Work out the finished part from the listing and answer in its coordinate system (mm). A direction names the side the tool comes from. Coordinates: 2 decimals unless noted, no trailing zeros. Order: outer loops, then holes, each group sorted by start corner. A loop starts at its lowest first (then second) coordinate and runs counter-clockwise, first axis right, second up. Notation, with made-up numbers: M -26,-16 L -14,-16 A17 cw -14,12 Z; hole C 74.25,-29 d9. An arc over 180 degrees is marked long. Answer in a Markdown table with one row per item. Add a question column.
Item 1: The part is cut by section B-B (x = 0). State how many separate pieces and enclosed holes the cut face has, then the cut area to 3 significant figures.
Item 2: Flat-ended cylindrical pins translate along their axes: pin 1 Ø0.8 at (x, y) = (0.5, 0) entering from +Z; pin 2 Ø2.5 at (x, z) = (-2.5, 1.5) entering from -Y; pin 3 Ø0.5 at (x, z) = (0.5, 19) entering from +Y; pin 4 Ø1 at (x, z) = (0, 19.32) entering from +Y. Find the tip coordinate at first contact, or state that the pin passes through.
Item 3: Consider line 1 (Y direction, x = 0, z = 16.2) (3 decimals); line 2 (Z direction, x = 0, y = 1); line 3 (Z direction, x = 0, y = 32.35). Determine where each line is inside the solid, lowest interval first. Write a range as from..to.
Item 4: Which of the six approach directions +Z, -Z, +X, -X, +Y, -Y give full straight-line access (tool end or side, diameter ignored) to faces 1 (the face through (-0.925, -0.5, -0.2)), 2 (the face through (0, 0.7, 13)), 3 (the face through (0, 15, 13.824)), 4 (the face through (0.925, -0.5, -0.2))?
Item 5: The mould has two halves that part along X. Classify faces 5 (the face through (-3.05, 2, 8)), 6 (the face through (0, 33.5, 18)), 7 (the face through (0.1, 1.17, 2.23)): released by +X, released by -X, zero draft, split by the parting line, or undercut.
Item 6: The part is cut by section C-C (y = 2). Write down the section's boundary in (x, z), then the cut area to 3 significant figures.
Item 7: The part is cut by section D-D (z = 10). Write down the section's boundary in (x, y).
Item 8: The part is cut by section A-A (z = -2.5). Write down the section's boundary in (x, y) (3 decimals), then the cut area to 3 significant figures.
Autodesk Inventor part; units mm, degrees
ref_plane "Work Plane3" through (-3.05, 3.4, 13.8245) normal (0, 0, 1) x (1, 0, 0)
ref_plane "YZ Plane" through (0, 0, 0) normal (1, 0, 0) x (0, 1, 0)
ref_plane "XZ Plane" through (0, 0, 0) normal (0, 1, 0) x (-1, 0, 0)
sketch "Sketch1" plane through (0, 0, 0) normal (0, 1, 0) x (-1, 0, 0)
  line L0 (3.05, -5.3255) -> (-3.05, -5.3255)
  line L1 (-3.05, -5.3255) -> (-3.05, 4.8245)
  line L2 (-3.05, 4.8245) -> (3.05, 4.8245)
  line L3 (3.05, 4.8245) -> (3.05, -5.3255)
  line L4 (0.925, 4.8245) -> (-0.925, 4.8245)
  line L5 (0.925, 4.8245) -> (0.925, -5.3255)
  line L6 (-0.925, 4.8245) -> (-0.925, -5.3255)
  circle A0 centre (0, 3.0245) radius 0.8
  circle A1 centre (0, -3.8255) radius 0.8
  line L7 (0, 4.8245) -> (0, -5.3255)
  line L8 (-3.05, 0) -> (3.05, 0)
  point P0 (0, 0)
  dimension "d13" = 6.1
  dimension "d44" = 1.85
  dimension "d45" = 2.125
  dimension "d46" = 1.6
  dimension "d47" = 1.6
  dimension "d128" = 6.85
extrude "Extrusion1" add sketch "Sketch1" along normal blind 3.4 contours L0 L5 L8 L3 | L0 L7 A1 L8 L5 | L8 L5 L2 L3 | L0 L6 L8 L7 A1 | L8 L7 A0 L2 L5 | L0 L1 L8 L6 | L8 L6 L2 L7 A0 | L8 L1 L2 L6
extrude "Extrusion6" add sketch "Sketch1" against normal blind 1 contours L0 L7 A1 L8 L5 | L0 L6 L8 L7 A1 | L8 L7 A0 L2 L5 | L8 L6 L2 L7 A0
sketch "Sketch13" plane through (-3.05, 3.4, 4.8245) normal (0, 0, 1) x (1, 0, 0)
  line L0 (0, 0) -> (0, -2.7)
  line L1 (0, -3.4) -> (0, 0)
  line L2 (0, -2.7) -> (6.1, -2.7)
  line L3 (6.1, -3.4) -> (6.1, 0)
  line L4 (6.1, 0) -> (6.1, -2.7)
  line L5 (0, 0) -> (6.1, 0)
  point P0 (3.05, -3.4)
  point P1 (6.1, -3.41)
  dimension "d56" = 2.7
extrude "Extrusion8" add sketch "Sketch13" along normal blind 17
sketch "Sketch17" plane through (-3.05, 3.4, 21.8245) normal (0, 0, 1) x (1, 0, 0)
  line L0 (6.1, 0) -> (0, 0)
  line L1 (6.1, 0) -> (19.567, 0) construction
  line L2 (16.968, 8.2706) -> (10.0894, 18.4685)
  line L3 (10.0894, 18.4685) -> (13.5713, 20.8172)
  line L4 (13.5713, 20.8172) -> (20.102, 11.1351)
  line L5 (20.102, 11.1351) -> (22.1374, 8.1174)
  line L6 (6.1, -3.4) -> (6.1, -2.7)
  line L7 (22.1374, 8.1174) -> (6.1, -2.7)
  line L8 (6.1, 0) -> (6.1, -2.7)
  line L9 (6.1, 0.94) -> (6.1, 0)
  line L10 (6.1, 0.94) -> (3.05, 0.94)
  line L11 (3.05, 0.94) -> (3.05, 0)
  line L12 (16.968, 8.2706) -> (6.1, 0.94)
  line L13 (6.1, 0.94) -> (7.7497, 0.94)
  point P0 (3.05, -3.4)
  dimension "d74" = 12.301
  dimension "d75" = 4.2
  dimension "d92" = 3.64
  dimension "d93" = 3.64
  dimension "d94" = 10.868
  dimension "d98" = 34
extrude "Extrusion12" [suppressed]
ref_plane "Work Plane3" through (-3.05, 3.4, 13.8245) normal (0, 0, 1) x (1, 0, 0)
sketch "Sketch29" plane through (-3.05, 3.4, 13.8245) normal (0, 0, 1) x (1, 0, 0)
  line L0 (3.85, -4.4) -> (2.25, -4.4)
  line L1 (3.05, -4.4) -> (3.05, 30.1)
  line L2 (4.95, 30.1) -> (3.05, 30.1)
  line L3 (3.05, 30.1) -> (1.15, 30.1)
  line L4 (6.1, -3.4) -> (6.1, 0)
  line L5 (4.95, 30.1) -> (6.1, 0)
  line L6 (0, -3.4) -> (0, 0)
  line L7 (1.15, 30.1) -> (0, 0)
  line L8 (0, 0) -> (6.1, 0)
  point P0 (3.05, -3.4)
  point P1 (3.0506, 28.6)
  dimension "d137" = 34.5
  dimension "d138" = 3.8
extrude "Extrusion20" add sketch "Sketch29" along normal blind 8
fillet "Fillet6" radius 0.5 2 edges at (2.475, 18.45, 13.8245) (-2.475, 18.45, 13.8245)
sketch "Sketch14" plane through (0, 3.4, 0) normal (0, 1, 0) x (1, 0, 0)
  line L0 (3.05, 5.3255) -> (3.05, -21.8245)
  line L1 (3.05, -21.8245) -> (3.05, -13.8245)
  line L2 (3.05, -13.8245) -> (-3.05, -13.8245)
  line L3 (-3.05, 5.3255) -> (-3.05, -21.8245)
  line L4 (-3.05, -21.8245) -> (3.05, -21.8245)
  point P0 (0, 0)
  dimension "d59" = 8
extrude "Extrusion9" [suppressed]
sketch "Sketch16" plane through (0, 35.4, 0) normal (0, 1, 0) x (1, 0, 0)
  circle A0 centre (-0.1175, -18.652) radius 1.5
  line L0 (1.9325, -20.707) -> (-1.9325, -20.707)
  line L1 (1.9325, -14.9419) -> (1.9325, -20.707)
  point P0 (0, 0)
  point P1 (0, -20.707)
  dimension "d67" = 3
  dimension "d68" = 2.055
  dimension "d69" = 2.05
extrude "Extrusion11" [suppressed]
sketch "Sketch15" plane through (-3.05, 3.4, 21.8245) normal (0, 0, 1) x (1, 0, 0)
  line L0 (2.6762, 10.6502) -> (2.7739, 7.8519) construction
  line L1 (6.1, 0) -> (4.9825, 32)
  line L2 (1.6768, 10.6153) -> (1.7746, 7.817)
  line L3 (3.7733, 7.8868) -> (3.6756, 10.6851)
  arc A0 (3.6756, 10.6851) -> (1.6768, 10.6153) centre (2.6762, 10.6502) ccw
  arc A1 (1.7746, 7.817) -> (3.7733, 7.8868) centre (2.7739, 7.8519) ccw
  point P0 (3.05, -3.4)
  point P1 (2.7251, 9.251)
  dimension "d62" = 1.4
  dimension "d63" = 2
  dimension "d64" = 3.05
extrude "Extrusion10" [suppressed]
sketch "Sketch20" plane through (10.5213, 24.2172, 21.8245) normal (-0.5591929, 0.8290376, 0) x (0.8290376, 0.5591929, 0)
  circle A0 centre (-2.15, 2.0494) radius 1.5
  line L0 (-4.2, 0) -> (-4.2, 4.1)
  line L1 (0, 0) -> (-4.2, 0)
  point P0 (-22.2646, 21.8245)
  point P1 (-2.1, 0)
  dimension "d82" = 3
  dimension "d83" = 2.05
  dimension "d84" = 2.05
extrude "Extrusion14" [suppressed]
sketch "Sketch18" plane through (-3.05, 3.4, 21.8245) normal (0, 0, 1) x (1, 0, 0)
  line L0 (12.7441, 18.3775) -> (14.3099, 16.0562) construction
  line L1 (11.9151, 17.8183) -> (13.4808, 15.497)
  line L2 (15.1389, 16.6154) -> (13.5732, 18.9367)
  arc A0 (13.5732, 18.9367) -> (11.9151, 17.8183) centre (12.7441, 18.3775) ccw
  arc A1 (13.4808, 15.497) -> (15.1389, 16.6154) centre (14.3099, 16.0562) ccw
  line L3 (22.1374, 8.1174) -> (13.5713, 20.8172)
  line L4 (10.0894, 18.4685) -> (13.5713, 20.8172)
  point P0 (3.05, -3.4)
  point P1 (13.527, 17.2169)
  point P2 (12.1849, 19.2066)
  dimension "d78" = 1.4
  dimension "d79" = 2
  dimension "d89" = 0.56
  dimension "d90" = 2.05
extrude "Extrusion13" [suppressed]
sketch "Sketch21" plane through (13.7716, 15.5536, 19.7751) normal (-0.5591929, 0.8290376, 0) x (0.8290376, 0.5591929, 0)
  circle A0 centre (0, 0) radius 0.868
  point P0 (-20.1146, 19.7751)
extrude "Extrusion15" [suppressed]
mirror "Mirror3" [suppressed]
chamfer "Chamfer1" [suppressed]
fillet "Fillet1" [suppressed]
sketch "Sketch24" plane through (-3.05, 0, -5.3255) normal (-1, 0, 0) x (0, 0, 1)
  circle A0 centre (22.6257, 31.1455) radius 0.8
  point P0 (5.3255, 0)
  point P1 (27.15, 0.7)
  dimension "d109" = 1.6
extrude "Extrusion18" cut sketch "Sketch24" against normal through all
sketch "Sketch26" plane through (0, 35.4, 0) normal (0, 1, 0) x (1, 0, 0)
  circle A0 centre (0, -19.1945) radius 0.8
  point P0 (0, 0)
  dimension "d131" = 1.6
extrude "Extrusion19" [suppressed]
fillet "Fillet4" [suppressed]
sketch "Sketch31" plane through (-3.05, 3.4, 13.8245) normal (0, 0, -1) x (-1, 0, 0)
  line L0 (-3.05, -3.4) -> (-3.05, 28.5)
  circle A0 centre (-3.05, 28.5) radius 0.355
  dimension "d145" = 31.9
  dimension "d147" = 0.71
extrude "Extrusion22" cut sketch "Sketch31" against normal through all
sketch "Sketch33" plane through (-1.9, 33.5, 21.8245) normal (0, 1, 0) x (1, 0, 0)
  line L0 (3.8, 0) -> (0, 0)
  line L1 (3.8, 7.5) -> (3.8, 0)
  line L2 (0, 7.5) -> (0, 0)
  circle A0 centre (1.9, 2.5) radius 0.8
  line L3 (1.9, 2.5) -> (3.8, 2.5)
  line L4 (1.9, 2.5) -> (0, 2.5)
  point P0 (1.9, 21.8245)
  dimension "d150" = 1.6
  dimension "d151" = 2.5
extrude "Extrusion23" cut sketch "Sketch33" against normal blind 2 contours L3 L4 A0 | A0 L4 L3
fillet "Fillet7" radius 0.5 4 edges at (-1.9, 33.5, 18.0745) (1.7534, 33.5, 13.9709) (0, 33.5, 13.8245) (1.9, 33.5, 18.0745)
sketch "Sketch34" plane through (-3.05, 3.4, 13.8245) normal (0, 0, -1) x (-1, 0, 0)
  point P0 (-3.05, -3.4)
equation "\"d13\" = base_width"
equation "\"d45\" = -0.5 * d44 + 0.5 * d13"
equation "\"d4\" = base_length"
equation "\"base_width\" = 6.1"
equation "\"base_length\" = 3.4"
equation "\"base_screw_diameter\" = 1.5"
equation "\"base_screw_spacing_edge\" = 8.5"
equation "\"multi_angle\" = 34deg"
properties part number "microstim_holder_bottom"
Reply:
| question | item | result |
|---|---|---|
| 1 | separate pieces | 5 |
| 1 | enclosed holes | 0 |
| 1 | area | 308 mm2 |
| 2 | pin 1 | stops at z = 4.82 |
| 2 | pin 2 | stops at y = 0 |
| 2 | pin 3 | stops at y = 33.5 |
| 2 | pin 4 | stops at y = 31.5 |
| 3 | line 1 | y = 0.7..31.545, 32.255..33.5 |
| 3 | line 2 | z = -5.33..-4.63, -3.03..2.22, 3.82..21.82 |
| 3 | line 3 | z = 13.82..18.52, 20.12..21.82 |
| 4 | face 1 | +Z, -Z, -X, -Y |
| 4 | face 2 | +Z, +X, -X, -Y |
| 4 | face 3 | -Z, +X, -X, +Y |
| 4 | face 4 | +Z, -Z, +X, -Y |
| 5 | face 5 | released by -X |
| 5 | face 6 | zero draft |
| 5 | face 7 | undercut |
| 6 | outline | M -3.05,-5.33 L 3.05,-5.33 L 3.05,21.82 L -3.05,21.82 Z; hole C 0,-3.83 d1.6; hole C 0,3.02 d1.6 |
| 6 | area | 162 mm2 |
| 7 | outline | M -3.05,0.7 L 3.05,0.7 L 3.05,3.4 L -3.05,3.4 Z |
| 8 | outline | M -3.05,0 L -0.925,0 L -0.925,-1 L 0.925,-1 L 0.925,0 L 3.05,0 L 3.05,3.4 L -3.05,3.4 Z |
| 8 | area | 22.6 mm2 |
